Could you check a few things on this model? Use its own coordinates, in mm. Face numbers are marked on the shaded views. Round coordinates to 2 decimals unless told otherwise and drop trailing zeros. Loops run counter-clockwise (first coordinate to the right, second up) from the corner with the lowest first, then second, coordinate; pieces in that order, holes last. Notation, with made-up numbers: (-8, -35) -> (8, -35) arc R15 cw to (8, -30) -> close; hole circle Ø9 at (11.25, 45). An arc over 180 degrees is marked (long way). One line per item, written item: value.
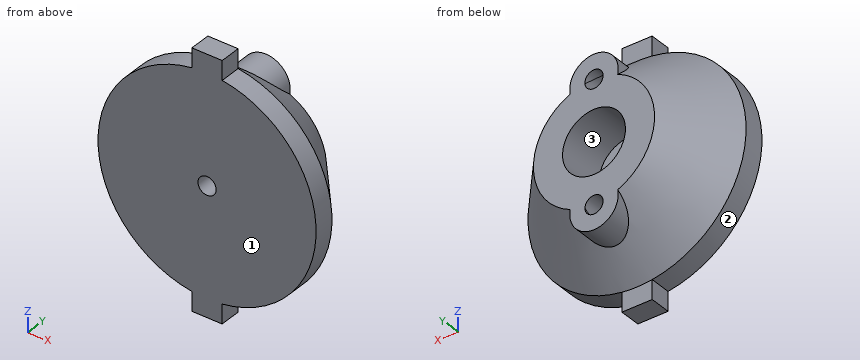
```python
from build123d import *

# Parameters (mm, degrees)
CROQUIS2_R                  = 4
CROQUIS2_R_2                = 1.5
SALIENTE_EXTRUIR1_DEPTH     = 10
CROQUIS3_R                  = 5.192385193
CROQUIS3_R_2                = 1.5
CORTAR_EXTRUIR1_DEPTH       = 8
CROQUIS4_W                  = 5
CROQUIS4_H                  = 42
SALIENTE_EXTRUIR2_DEPTH     = 3.5
SALIENTE_EXTRUIR3_START     = -5
SALIENTE_EXTRUIR3_OUTLINE_R = 1.5
SALIENTE_EXTRUIR3_DEPTH     = 5


# Read off the part's stored shape, not the designer's step: Saliente-Extruir3
with BuildPart() as part:
    # Croquis1 → Revolución1 (revolve)
    with BuildSketch(Plane.XY, mode=Mode.PRIVATE) as revoluci_n1_sk:
        Polygon((0, 0), (18, 0), (18, 3.5), (10, 13), (0, 13), align=None)
    revolve(revoluci_n1_sk.sketch.rotate(Axis((0, 0, 0), (0, 1, 0)), 90), axis=Axis((0, 0, 0), (0, 1, 0)))

    # Croquis2 → Saliente-Extruir1 (add)
    # profile 1 of 2: a face of its own
    with BuildSketch(Plane(origin=(0, 13, 0), x_dir=(1, 0, 0), z_dir=(0, 1, 0))):
        with Locations((0, 10)):
            Circle(CROQUIS2_R)
        with Locations((0, 10)):
            Circle(CROQUIS2_R_2, mode=Mode.SUBTRACT)
    # profile 2 of 2: a face of its own
    with BuildSketch(Plane(origin=(0, 13, 0), x_dir=(1, 0, 0), z_dir=(0, 1, 0))):
        with Locations((0, -10)):
            Circle(CROQUIS2_R)
        with Locations((0, -10)):
            Circle(CROQUIS2_R_2, mode=Mode.SUBTRACT)
    extrude(amount=-SALIENTE_EXTRUIR1_DEPTH)

    # Croquis3 → Cortar-Extruir1 (cut)
    with BuildSketch(Plane(origin=(0, 13, 0), x_dir=(1, 0, 0), z_dir=(0, 1, 0))):
        with Locations(Location((0, 0, 0), (0, 0, 270))):
            Circle(CROQUIS3_R)
        with Locations(Location((0, 10, 0), (0, 0, 270))):
            Circle(CROQUIS3_R_2)
        with Locations(Location((0, -10, 0), (0, 0, 270))):
            Circle(CROQUIS3_R_2)
    extrude(amount=-CORTAR_EXTRUIR1_DEPTH, mode=Mode.SUBTRACT)

    # Croquis4 → Saliente-Extruir2 (add)
    with BuildSketch(Plane.XZ):
        Rectangle(CROQUIS4_W, CROQUIS4_H)
    extrude(amount=-SALIENTE_EXTRUIR2_DEPTH)

    # Saliente-Extruir3 outline → Saliente-Extruir3 (cut)
    with BuildSketch(Plane(origin=(0, 5, 0), x_dir=(1, 0, 0), z_dir=(0, 1, 0)).offset(SALIENTE_EXTRUIR3_START)):
        Circle(SALIENTE_EXTRUIR3_OUTLINE_R)
    extrude(amount=SALIENTE_EXTRUIR3_DEPTH, mode=Mode.SUBTRACT)


solid = part.part
```
(1) We'd pull the mould along Z, two halves only. Please class the marked faces 1, 2 and 3: +Z half, -Z half, draft (parallel to the pull), parting line (faces both ways), or undercut.
Results below:
face 1: draft
face 2: parting line
face 3: undercut
(2) Please list where these lines run through material, in increasing order: L1, parallel to X at y = 2, z = 0; L2, parallel to Z at x = 0, y = 3.2; L3, parallel to X at y = 11.25, z = 10.
Results below:
L1: x = -18 to -1.5, 1.5 to 18
L2: z = -21 to -1.5, 1.5 to 21
L3: x = -5.63 to -1.5, 1.5 to 5.63
(3) Imagine slicing it at D-D on y = 6.5. Write out the boundary of the cut face in (x, z).
Results below:
outline: circle Ø30.95 at (0, 0); hole circle Ø10.38 at (0, 0); hole circle Ø3 at (0, -10); hole circle Ø3 at (0, 10)
(4) Imagine slicing it at C-C on y = 4.25. Write out the boundary of the cut face in (x, z), then the cut area to 3 significant figures.
Results below:
outline: circle Ø34.74 at (0, 0); hole circle Ø3 at (0, 0)
area: 941 mm²
(5) Imagine slicing it at B-B on z = 0. Write out the boundary of the cut face in (x, y), then the cut area to 3 significant figures.
Results below:
outline: (-18, 0) -> (-1.5, 0) -> (-1.5, 5) -> (-5.19, 5) -> (-5.19, 13) -> (-10, 13) -> (-18, 3.5) -> close; (1.5, 0) -> (18, 0) -> (18, 3.5) -> (10, 13) -> (5.19, 13) -> (5.19, 5) -> (1.5, 5) -> close
area: 294 mm²
(6) For pin 1 Ø1.6 at (y, z) = (2, -20) entering from -X; pin 2 Ø5 at (x, y) = (-9, 9.5) entering from -Z; pin 3 Ø1 at (x, z) = (-0.5, -19) entering from +Y, each with a flat end and sliding along its axis, tell me the tip position at first contact or that it passes through.
Results below:
pin 1: stops at x = -2.5
pin 2: stops at z = -12.58
pin 3: stops at y = 3.5
(7) Imagine slicing it at A-A on x = 0. Write out the boundary of the cut face in (y, z).
Results below:
outline: (0, -21) -> (3.5, -21) -> (3.5, -18) -> (8.25, -14) -> (13, -14) -> (13, -11.5) -> (5, -11.5) -> (5, -8.5) -> (13, -8.5) -> (13, -5.19) -> (5, -5.19) -> (5, -1.5) -> (0, -1.5) -> close; (0, 1.5) -> (5, 1.5) -> (5, 5.19) -> (13, 5.19) -> (13, 8.5) -> (5, 8.5) -> (5, 11.5) -> (13, 11.5) -> (13, 14) -> (8.25, 14) -> (3.5, 18) -> (3.5, 21) -> (0, 21) -> close
